```python
from build123d import *

# Parameters (mm, degrees)
SKETCH1_R           = 17.5
BOSS_EXTRUDE1_DEPTH = 24
SKETCH2_R           = 3.75
BOSS_EXTRUDE2_DEPTH = 3.5
SKETCH3_R           = 2.5
BOSS_EXTRUDE3_DEPTH = 16.5
CHAMFER1_SIZE       = 2.54
SKETCH5_R           = 17.5
BOSS_EXTRUDE4_DEPTH = 9.5
CHAMFER2_SIZE       = 2.54
SKETCH6_R           = 3
BOSS_EXTRUDE5_DEPTH = 1
SKETCH7_R           = 1
CUT_EXTRUDE1_DEPTH  = 25.4


with BuildPart() as part:
    # Sketch1 → Boss-Extrude1 (new body)
    with BuildSketch(Plane(origin=(0, 0, 0), x_dir=(1, 0, 0), z_dir=(0, 1, 0))):
        Circle(SKETCH1_R)
    extrude(amount=BOSS_EXTRUDE1_DEPTH)

    # Sketch2 → Boss-Extrude2 (add)
    with BuildSketch(Plane(origin=(0, 24, 0), x_dir=(1, 0, 0), z_dir=(0, 1, 0))):
        Circle(SKETCH2_R)
    extrude(amount=BOSS_EXTRUDE2_DEPTH)

    # Sketch3 → Boss-Extrude3 (add)
    with BuildSketch(Plane(origin=(0, 27.5, 0), x_dir=(1, 0, 0), z_dir=(0, 1, 0))):
        Circle(SKETCH3_R)
    extrude(amount=BOSS_EXTRUDE3_DEPTH)

    # Chamfer1
    chamfer1_edges = [part.edges().sort_by_distance(p)[0] for p in [
        (-17.5, 24, 0),
    ]]
    chamfer(chamfer1_edges, length=CHAMFER1_SIZE)

    # Sketch5 → Boss-Extrude4 (add)
    with BuildSketch(Plane.XZ):
        Circle(SKETCH5_R)
    extrude(amount=BOSS_EXTRUDE4_DEPTH)

    # Chamfer2
    chamfer2_edges = [part.edges().sort_by_distance(p)[0] for p in [
        (-17.5, -9.5, 0),
    ]]
    chamfer(chamfer2_edges, length=CHAMFER2_SIZE)

    # Sketch6 → Boss-Extrude5 (add)
    with BuildSketch(Plane.XZ.offset(9.5)):
        Circle(SKETCH6_R)
    extrude(amount=BOSS_EXTRUDE5_DEPTH)

    # Sketch7 → Cut-Extrude1 (cut)
    with BuildSketch(Plane(origin=(0, 24, 0), x_dir=(1, 0, 0), z_dir=(0, 1, 0))):
        with Locations((0, 9.5)):
            Circle(SKETCH7_R)
        with Locations((12.5, 0)):
            Circle(SKETCH7_R)
        with Locations((0, -9.5)):
            Circle(SKETCH7_R)
        with Locations((-12.5, 0)):
            Circle(SKETCH7_R)
    extrude(amount=-CUT_EXTRUDE1_DEPTH, mode=Mode.SUBTRACT)


solid = part.part
```
The listing builds one solid part. Answer for the finished solid, in the listing's coordinates (mm). A direction names the side the tool comes from. Round coordinates to 2 decimals unless told otherwise and drop trailing zeros. Loops run counter-clockwise (first coordinate to the right, second up) from the corner with the lowest first, then second, coordinate; pieces in that order, holes last.
1) Consider line 1 (X direction, y = 6.25, z = 0); line 2 (Y direction, x = -7.5, z = -4.5); line 3 (X direction, y = 10.5, z = 9.5). Determine where each line is inside the solid, lowest interval first.
Outcome:
line 1: x = -17.5 to -13.5, -11.5 to 11.5, 13.5 to 17.5
line 2: y = -9.5 to 24
line 3: x = -14.7 to -1, 1 to 14.7
2) A cutting plane is placed at A-A on y = 16. Determine the outline of the cut face in (x, z).
Outcome:
outline: circle Ø35 at (0, 0); hole circle Ø2 at (-12.5, 0); hole circle Ø2 at (0, -9.5); hole circle Ø2 at (0, 9.5); hole circle Ø2 at (12.5, 0)
3) Given P1, Ø1.6, axis at x = -12.5, z = 0, coming from the -Y side; P2, Ø1, axis at x = 8, y = 23, coming from the -Z side; P3, Ø2, axis at x = 11, y = -2, coming from the +Z side, each flat-ended and moving along its own axis, determine where each tip first touches the part or whether it passes through.
Outcome:
P1: stops at y = -9.5
P2: stops at z = -14.45
P3: stops at z = 14.36
4) A cutting plane is placed at C-C on y = -3.5. Determine the outline of the cut face in (x, z), plus the area to 3 significant figures.
Outcome:
outline: circle Ø35 at (0, 0)
area: 962 mm2
5) A cutting plane is placed at B-B on x = 0. Determine the outline of the cut face in (y, z).
Outcome:
outline: (-10.5, -3) - (-9.5, -3) - (-9.5, -14.96) - (-6.96, -17.5) - (21.46, -17.5) - (24, -14.96) - (24, -10.5) - (-1.4, -10.5) - (-1.4, -8.5) - (24, -8.5) - (24, -3.75) - (27.5, -3.75) - (27.5, -2.5) - (44, -2.5) - (44, 2.5) - (27.5, 2.5) - (27.5, 3.75) - (24, 3.75) - (24, 8.5) - (-1.4, 8.5) - (-1.4, 10.5) - (24, 10.5) - (24, 14.96) - (21.46, 17.5) - (-6.96, 17.5) - (-9.5, 14.96) - (-9.5, 3) - (-10.5, 3) - close
6) For a pull along Z with two mould halves and no side action, classify faces 1 (the face through (-0.13, 11.48, 8.51)), 2 (the face through (12, -1.4, 0)), 3 (the face through (-11.97, -9.377, -9.178)), 4 (the face through (3, 24, 3)) as released by +Z, released by -Z, zero draft, split by the parting line, or undercut.
Outcome:
face 1: undercut
face 2: undercut
face 3: split by the parting line
face 4: zero draft
7) A cutting plane is placed at D-D on y = 32.5. Determine the outline of the cut face in (x, z).
Outcome:
outline: circle Ø5 at (0, 0)
8) For faces 5 (the face through (0, -10.5, 0)), 6 (the face through (-13, -1.4, 0)), 7 (the face through (-3, -10, 0)), determine the directions among +Z, -Z, +X, -X, +Y, -Y from which every point of the face is accessible in a straight line to the end or side of a thin tool.
Outcome:
face 5: +Z, -Z, +X, -X, -Y
face 6: +Y
face 7: -Y
